Input: part model. Units: mm. Frame: model coordinates. Give positions to 0.01 mm unless a question says otherwise; leave off trailing zeros. Write each loop counter-clockwise with the first axis right and the second up, starting at its lowest first coordinate (ties: lowest second). Pieces come first, ordered by that corner, then holes. Notation, with made-up numbers: M -35.75,63.5 L 22.25,63.5 A18 ccw 22.25,98.5 Z; hole C -23,82.5 d9. An arc over 180 degrees is marked long. Use CSV: the item, a comma, the result in double quotes. Start each with the question number.
from build123d import *

# Parameters (mm, degrees)
BOSS_EXTRUDE1_DEPTH = 4.826
BOSS_EXTRUDE2_DEPTH = 5.08
BOSS_EXTRUDE2_TAPER = 5


with BuildPart() as part:
    # Sketch1 → Boss-Extrude1 (new body)
    with BuildSketch(Plane.XY):
        with BuildLine():
            Line((-0.385, -1.9725), (0.385, -1.9725))
            ThreePointArc((0.385, -1.9725), (1.507532015, -1.507532015), (1.9725, -0.385))
            Line((1.9725, -0.385), (1.9725, 0.385))
            ThreePointArc((1.9725, 0.385), (1.507532015, 1.507532015), (0.385, 1.9725))
            Line((0.385, 1.9725), (-0.385, 1.9725))
            ThreePointArc((-0.385, 1.9725), (-1.507532015, 1.507532015), (-1.9725, 0.385))
            Line((-1.9725, 0.385), (-1.9725, -0.385))
            ThreePointArc((-1.9725, -0.385), (-1.507532015, -1.507532015), (-0.385, -1.9725))
        make_face()
    boss_extrude1 = extrude(amount=BOSS_EXTRUDE1_DEPTH)

    # Sketch2 → Boss-Extrude2 (add)
    with BuildSketch(Plane.XY.offset(4.826)):
        with BuildLine():
            Line((1.9725, -0.385), (1.9725, 0.385))
            ThreePointArc((1.9725, 0.385), (1.507532015, 1.507532015), (0.385, 1.9725))
            Line((0.385, 1.9725), (-0.385, 1.9725))
            ThreePointArc((-0.385, 1.9725), (-1.507532015, 1.507532015), (-1.9725, 0.385))
            Line((-1.9725, 0.385), (-1.9725, -0.385))
            ThreePointArc((-1.9725, -0.385), (-1.507532015, -1.507532015), (-0.385, -1.9725))
            Line((-0.385, -1.9725), (0.385, -1.9725))
            ThreePointArc((0.385, -1.9725), (1.507532015, -1.507532015), (1.9725, -0.385))
        make_face()
    boss_extrude2 = extrude(amount=BOSS_EXTRUDE2_DEPTH, taper=BOSS_EXTRUDE2_TAPER)

    # Mirror1: Boss-Extrude1, Boss-Extrude2 across plane
    add(boss_extrude1.mirror(Plane.XY))
    add(boss_extrude2.mirror(Plane.XY))


solid = part.part
Q1. Section A-A, the plane z = -2. Return the cut outline in (x, y) (1 decimal), and give its area (3 significant figures).
Q2. First-contact query: pin 1 Ø1 at (x, z) = (-1.5, -6) entering from +Y; pin 2 Ø1 at (x, z) = (-1.5, -1.5) entering from +Y; pin 3 Ø1.5 at (y, z) = (1.5, -0.5) entering from +X. Flat tips, straight axial feed; report the tip coordinate or a pass-through.
Q3. Section B-B, the plane y = -0.15. Return the cut outline in (x, z).
Q4. Material intervals for L1, parallel to X at y = -0.5, z = -7.5; L2, parallel to Y at x = 1.15, z = -2.25; L3, parallel to X at y = 0.75, z = 5.25, sorted ascending. Write a range as [from, to].
Check result:
1,outline,"M -2,-0.4 A1.6 ccw -0.4,-2 L 0.4,-2 A1.6 ccw 2,-0.4 L 2,0.4 A1.6 ccw 0.4,2 L -0.4,2 A1.6 ccw -2,0.4 Z"
1,area,"13.4 mm²"
2,pin 1,"stops at y = 1.74"
2,pin 2,"stops at y = 1.85"
2,pin 3,"stops at x = 1.93"
3,outline,"M -1.97,-4.83 L -1.53,-9.91 L 1.53,-9.91 L 1.97,-4.83 L 1.97,4.83 L 1.53,9.91 L -1.53,9.91 L -1.97,4.83 Z"
4,L1,"x = [-1.73, 1.73]"
4,L2,"y = [-1.78, 1.78]"
4,L3,"x = [-1.89, 1.89]"
